Autodesk Inventor part; units mm, degrees
ref_plane "YZ Plane" through (0, 0, 0) normal (1, 0, 0) x (0, 1, 0)
ref_plane "XZ Plane" through (0, 0, 0) normal (0, 1, 0) x (-1, 0, 0)
ref_plane "XY Plane" through (0, 0, 0) normal (0, 0, 1) x (1, 0, 0)
sketch "Sketch1" plane through (0, 0, 0) normal (0, 1, 0) x (-1, 0, 0)
  line L0 (0, 0) -> (10, 0)
  line L1 (10, 0) -> (10, -112)
  line L2 (10, -112) -> (0, -112)
  line L3 (0, -112) -> (0, 0)
  line L4 (10, -112) -> (10, -147)
  line L5 (10, -147) -> (30, -147)
  line L6 (10, 0) -> (10, 35)
  line L7 (10, 35) -> (30, 35)
  line L8 (30, 35) -> (30, -147)
  dimension "d16" = 35
  dimension "d17" = 20
  dimension "d18" = 35
  dimension "d19" = 20
  dimension "d28" = 112
  dimension "d35" = 10
extrude "Extrusion1" add sketch "Sketch1" along normal blind 30
sketch "Sketch2" plane through (0, 0, 0) normal (0, -1, 0) x (1, 0, 0)
  line L0 (-30, -147) -> (-30, 35)
  line L1 (-30, -96) -> (-10, -96)
  line L2 (-10, -96) -> (-10, -16)
  line L3 (-10, -16) -> (-30, -16)
  line L4 (-30, -16) -> (-30, -96)
  line L5 (-10, 0) -> (0, 0)
  dimension "d22" = 20
  dimension "d23" = 80
  dimension "d25" = 16
extrude "Extrusion2" cut sketch "Sketch2" against normal blind 10
sketch "Sketch3" plane through (0, 0, 0) normal (0, -1, 0) x (1, 0, 0)
  line L0 (-10, -16) -> (-10, -96)
  line L1 (-10, -96) -> (-20, -96)
  line L2 (-20, -96) -> (-20, -147)
  line L3 (-20, -147) -> (-10, -147)
  line L4 (-10, -147) -> (-10, -96)
  line L5 (-10, -16) -> (-20, -16)
  line L6 (-20, -16) -> (-20, 35)
  line L7 (-20, 35) -> (-10, 35)
  line L8 (-10, 35) -> (-10, -16)
  point P0 (0, 0)
  dimension "d29" = 10
  dimension "d30" = 51
  dimension "d31" = 10
  dimension "d32" = 51
extrude "Extrusion3" add sketch "Sketch3" along normal blind 90
properties part number "CatwalkHolder"
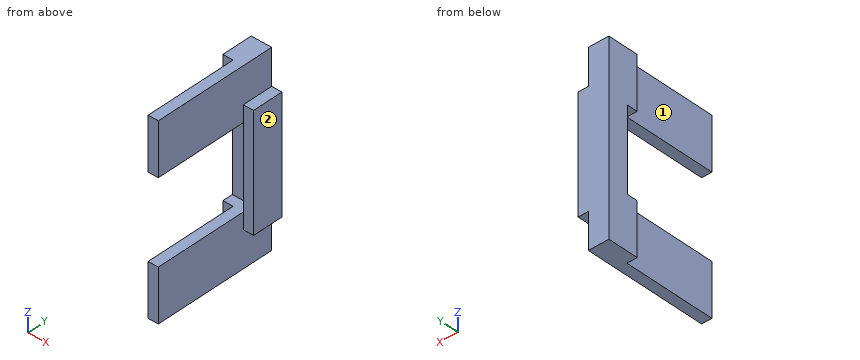
Part model, mm, in its own coordinate system. Face numbers are marked on the shaded views. A direction names the side the tool comes from. Give positions to 0.01 mm unless a question says otherwise; leave off trailing zeros. Write each loop counter-clockwise with the first axis right and the second up, starting at its lowest first coordinate (ties: lowest second). Pieces come first, ordered by that corner, then holes. Notation, with made-up numbers: (36.5, 86) -> (55.5, 86) arc R21 cw to (55.5, 122) -> close; hole circle Ø3 at (-6.75, 4.5). An arc over 180 degrees is marked (long way). Put each result on its own line as item: value. Start each with the question number.
Item 1: Cut at C-C (z = -63). List the corners of the cut face in (x, y).
Item 2: Which spindle directions (+Z, -Z, +X, -X, +Y, -Y) get a long thin tool onto all of the face, cutting with end or side? Do the marked faces 1 and 2. Say none if no direction does.
Item 3: Cut at B-B (x = -13.75). List the corners of the cut face in (y, z).
Item 4: Pin check, flat tips, straight feed: pin 1 Ø12 at (y, z) = (-71, 7) entering from -X; pin 2 Ø8 at (y, z) = (5.5, -52) entering from -X; pin 3 Ø5 at (x, z) = (-27, -121.5) entering from -Y. Stop position of each tip, or through.
Item 5: Cut at A-A (y = -2.5). List the corners of the cut face in (x, z), then the cut area to 3 significant figures.
Item 6: Wall check: L1, parallel to Z at x = -14.25, y = 4.5; L2, parallel to X at y = 23, z = 11; L3, parallel to X at y = -66, z = -113. Give the ranges that are in metal, low to high. Write a range as [from, to].
Item 7: Cut at D-D (y = 16.5). List the corners of the cut face in (x, z), then the cut area to 3 significant figures.
Answer list:
1. outline: (-30, 10) -> (-10, 10) -> (-10, 0) -> (0, 0) -> (0, 30) -> (-30, 30) -> close
2. face 1: +Z, -Z, -X, -Y
2. face 2: +Z, -Z, +X, +Y, -Y
3. outline: (-90, -147) -> (30, -147) -> (30, 35) -> (-90, 35) -> (-90, -16) -> (10, -16) -> (10, -96) -> (-90, -96) -> close
4. pin 1: stops at x = -20
4. pin 2: stops at x = -10
4. pin 3: stops at y = 0
5. outline: (-20, -147) -> (-10, -147) -> (-10, -96) -> (-20, -96) -> close; (-20, -16) -> (-10, -16) -> (-10, 35) -> (-20, 35) -> close
5. area: 1,020 mm2
6. L1: z = [-147, -96], [-16, 35]
6. L2: x = [-30, -10]
6. L3: x = [-20, -10]
7. outline: (-30, -147) -> (-10, -147) -> (-10, -112) -> (0, -112) -> (0, 0) -> (-10, 0) -> (-10, 35) -> (-30, 35) -> close
7. area: 4,760 mm2
